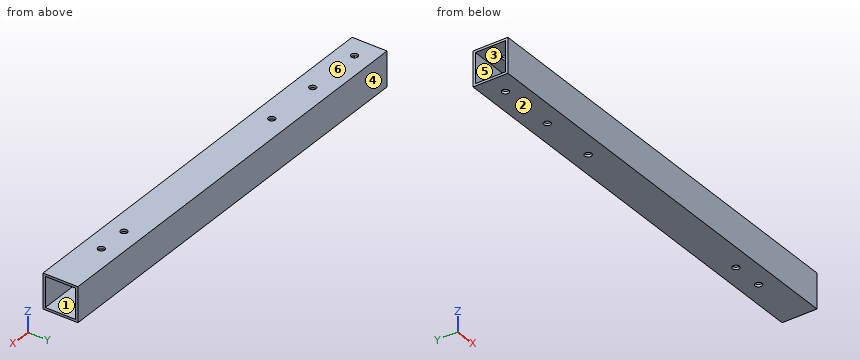
```python
from build123d import *

# Parameters (mm, degrees)
SKETCH_1_W          = 15
SKETCH_1_H          = 15
SKETCH_1_W_2        = 13
SKETCH_1_H_2        = 13
EXTRUDE_1_DEPTH     = 185
SKETCH_2_R          = 1.45
CUT_EXTRUDE_1_DEPTH = 186.758579883


with BuildPart() as part:
    # 草图1 → 凸台-拉伸1 (new body)
    with BuildSketch(Plane(origin=(0, 0, 0), x_dir=(0, 0, -1), z_dir=(1, 0, 0))):
        Rectangle(SKETCH_1_W, SKETCH_1_H)
        Rectangle(SKETCH_1_W_2, SKETCH_1_H_2, mode=Mode.SUBTRACT)
    extrude(amount=EXTRUDE_1_DEPTH)

    # 草图2 → 切除-拉伸1 (cut, through all)
    with BuildSketch(Plane(origin=(0, 0, -7.5), x_dir=(-1, 0, 0), z_dir=(0, 0, -1))):
        with Locations((-9.010396093, 0)):
            Circle(SKETCH_2_R)
        with Locations((-160.5, 0)):
            Circle(SKETCH_2_R)
        with Locations((-147, 0)):
            Circle(SKETCH_2_R)
        with Locations((-58.5, 0)):
            Circle(SKETCH_2_R)
        with Locations((-34.010396093, 0)):
            Circle(SKETCH_2_R)
    extrude(amount=-CUT_EXTRUDE_1_DEPTH, mode=Mode.SUBTRACT)


solid = part.part
```
Input: part model. Units: mm. Frame: model coordinates. Face numbers are marked on the shaded views. A direction names the side the tool comes from. Coordinates: 2 decimals unless noted, no trailing zeros. Write each loop counter-clockwise with the first axis right and the second up, starting at its lowest first coordinate (ties: lowest second). Pieces come first, ordered by that corner, then holes. Notation, with made-up numbers: (-30, 83.5) - (29, 83.5) arc R13 cw to (29, 92.5) - close; hole circle Ø7 at (27, -9.5). An arc over 180 degrees is marked (long way). Put each result on its own line as item: value. Start each with the question number.
1) Cut plane C-C (x = 154.5). Return the cut outline in (y, z), plus the area to 3 significant figures.
2) Cut plane A-A (y = 4.5). Return the cut outline in (x, z), plus the area to 3 significant figures.
3) Mould query, pull axis Z, two halves, no side actions, for the marked faces 1, 2, 3 and 4. Classes: pulls with the +Z half, pulls with the -Z half, needs draft (parallel to the pull), parting line crosses it, or undercut.
4) Ray query, L1, parallel to Y at x = 171.5, z = 5; L2, parallel to Y at x = 147, z = -7.05. Return the intervals inside material, ascending.
5) Reachability of the marked faces 5 and 6 from +Z, -Z, +X, -X, +Y, -Y: full face, straight path, thin tool, end or side. Return the list, or none.
Resolved:
1. outline: (-7.5, -7.5) - (7.5, -7.5) - (7.5, 7.5) - (-7.5, 7.5) - close; hole (-6.5, -6.5) - (6.5, -6.5) - (6.5, 6.5) - (-6.5, 6.5) - close
1. area: 56.0 mm2
2. outline: (0, -7.5) - (185, -7.5) - (185, -6.5) - (0, -6.5) - close; (0, 6.5) - (185, 6.5) - (185, 7.5) - (0, 7.5) - close
2. area: 370 mm2
3. face 1: undercut
3. face 2: pulls with the -Z half
3. face 3: undercut
3. face 4: needs draft
4. L1: y = -7.5 to -6.5, 6.5 to 7.5
4. L2: y = -7.5 to -1.45, 1.45 to 7.5
5. face 5: +X, -X
5. face 6: +Z, +X, -X, +Y, -Y
